Check sheet for the drawn part. Datum: minimum x, y, z corner. Units: mm. A direction names the side the tool comes from. Coordinates: 2 decimals unless noted, no trailing zeros. Write each loop counter-clockwise with the first axis right and the second up, starting at its lowest first coordinate (ties: lowest second). Pieces come first, ordered by that corner, then holes. Notation, with made-up numbers: (71, -11.5) - (77, -11.5) arc R29 cw to (77, 8.5) - close; hole circle Ø7 at (8, 19.5). An arc over 180 degrees is marked (long way). Use one line per item in the form item = value. Start each with the question number.
1. Scan lines: line 1 along Z through (x, y) = (7.5, 11); line 2 along Z through (x, y) = (11.5, 4); line 3 along Y through (x, z) = (2.5, 6). Record each from-to range of solid material in increasing order.
2. Cross-section at A-A on x = 10.75. Record the boundary of the cut face in (y, z).
3. Draft check along X on the marked faces 1, 2 and 3. Enter one of: +X half, -X half, draft (parallel to the pull), parting line (faces both ways), or undercut.
4. Go/stop test with flat-tipped pins: pin 1 Ø5.5 at (x, y) = (9, 6) entering from -Z; pin 2 Ø2 at (y, z) = (11.5, 15) entering from -X; pin 3 Ø5.5 at (y, z) = (6.5, 9) entering from +X; pin 4 Ø1.7 at (y, z) = (7, 22) entering from +X. Record where each tip stops, or that it passes through.
5. Cross-section at B-B on y = 10.25. Record the boundary of the cut face in (x, z).
6. Cross-section at C-C on z = 10.5. Record the boundary of the cut face in (x, y), then the cut area to 3 significant figures.
7. Tool access check on the marked faces 4, 5, 6, 7 and 8. Record the directions out of +Z, -Z, +X, -X, +Y, -Y that give a thin tool (end or side, any length) a straight path to the whole face; none if there is none.
8. Cross-section at D-D on x = 3.75. Record the boundary of the cut face in (y, z).
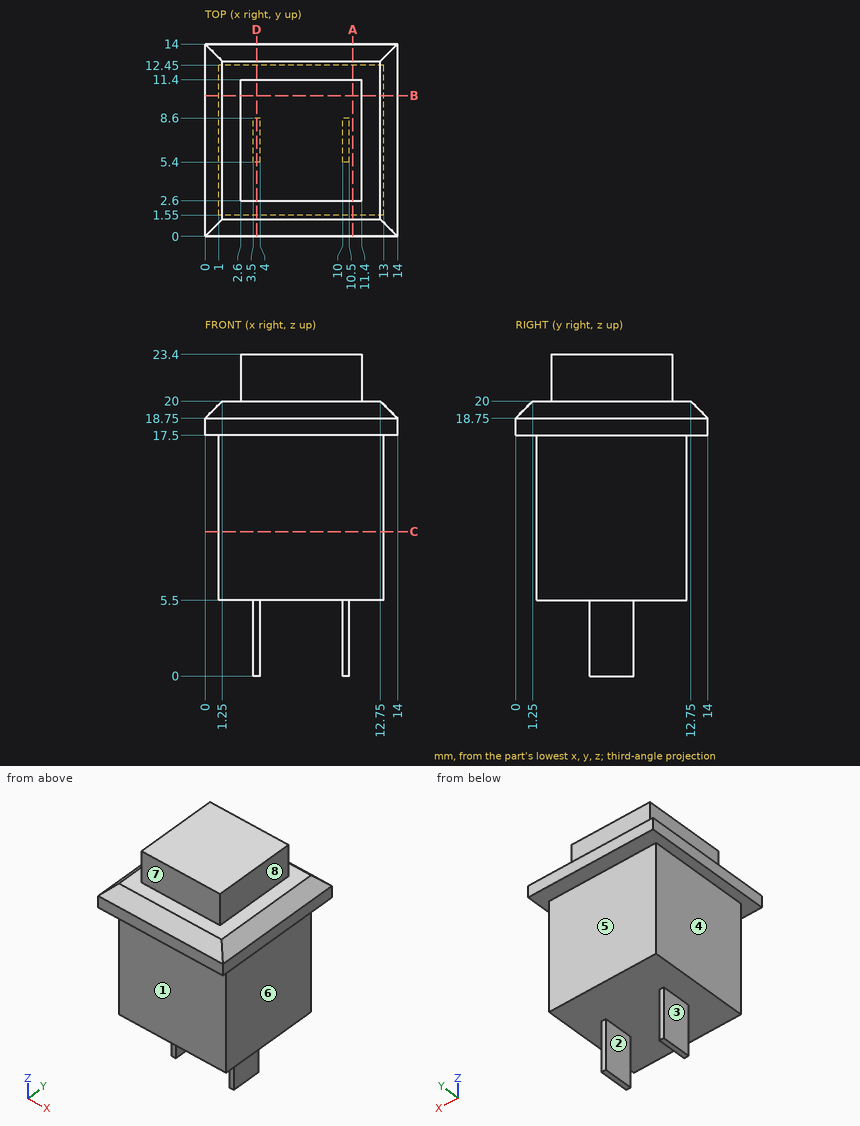
Final values:
q1.line_1 = 5.5 to 23.4
q1.line_2 = 5.5 to 20
q1.line_3 = 1.55 to 12.45
q2.outline = (0, 17.5) - (1.55, 17.5) - (1.55, 5.5) - (12.45, 5.5) - (12.45, 17.5) - (14, 17.5) - (14, 18.75) - (12.75, 20) - (11.4, 20) - (11.4, 23.4) - (2.6, 23.4) - (2.6, 20) - (1.25, 20) - (0, 18.75) - close
q3.face_1 = draft
q3.face_2 = undercut
q3.face_3 = -X half
q4.pin_1 = 0
q4.pin_2 = 1
q4.pin_3 = 13
q4.pin_4 = 11.4
q5.outline = (0, 17.5) - (1, 17.5) - (1, 5.5) - (13, 5.5) - (13, 17.5) - (14, 17.5) - (14, 18.75) - (12.75, 20) - (11.4, 20) - (11.4, 23.4) - (2.6, 23.4) - (2.6, 20) - (1.25, 20) - (0, 18.75) - close
q6.outline = (1, 1.55) - (13, 1.55) - (13, 12.45) - (1, 12.45) - close
q6.area = 131 mm²
q7.face_4 = -Z, -X, +Y, -Y
q7.face_5 = -Z, +X, -X, +Y
q7.face_6 = -Z, +X, +Y, -Y
q7.face_7 = +Z, +X, -X, -Y
q7.face_8 = +Z, +X, +Y, -Y
q8.outline = (0, 17.5) - (1.55, 17.5) - (1.55, 5.5) - (5.4, 5.5) - (5.4, 0) - (8.6, 0) - (8.6, 5.5) - (12.45, 5.5) - (12.45, 17.5) - (14, 17.5) - (14, 18.75) - (12.75, 20) - (11.4, 20) - (11.4, 23.4) - (2.6, 23.4) - (2.6, 20) - (1.25, 20) - (0, 18.75) - close
